Source: CAD feature listing. Evaluate the final solid. Frame: model axes, mm. Face numbers are marked on the shaded views. A direction names the side the tool comes from. Give positions to 0.01 mm unless a question says otherwise; leave off trailing zeros. Write each loop counter-clockwise with the first axis right and the second up, starting at its lowest first coordinate (ties: lowest second). Pieces come first, ordered by that corner, then holes. Notation, with made-up numbers: (31.25, 43) - (83.25, 43) arc R24 ccw to (83.25, 66) - close; hole circle Ø7 at (52, -11). An arc over 180 degrees is marked (long way). Answer as a JSON object with one key per item and string values. Group by question number.
from build123d import *

# Parameters (mm, degrees)
SKETCH1_R           = 10.85
SKETCH1_R_2         = 1.55
BOSS_EXTRUDE1_DEPTH = 7
CUT_EXTRUDE1_DEPTH  = 10
SKETCH3_R           = 1.55
BOSS_EXTRUDE2_DEPTH = 2.5
SKETCH6_W           = 5.995922228
SKETCH6_H           = 11.403727684
CUT_EXTRUDE3_DEPTH  = 11.5
CHAMFER2_SIZE       = 1
SKETCH7_R           = 1.5
CUT_EXTRUDE4_DEPTH  = 11.5
CHAMFER3_SIZE       = 0.5


with BuildPart() as part:
    # Sketch1 → Boss-Extrude1 (new body)
    with BuildSketch(Plane.XY):
        Circle(SKETCH1_R)
        with Locations((-7.8, 0)):
            Circle(SKETCH1_R_2, mode=Mode.SUBTRACT)
        with Locations(Location((7.8, 0, 0), (0, 0, 180))):
            Circle(SKETCH1_R_2, mode=Mode.SUBTRACT)
    extrude(amount=BOSS_EXTRUDE1_DEPTH)

    # Sketch2 → Cut-Extrude1 (cut)
    with BuildSketch(Plane.XY.offset(7)):
        with BuildLine():
            Line((-2.214560219, -5.749305929), (-2.214560219, -7.027203312))
            ThreePointArc((-2.214560219, -7.027203312), (-1.775220391, -8.087863484), (-0.714560219, -8.527203312))
            Line((-0.714560219, -8.527203312), (0.714560219, -8.527203312))
            ThreePointArc((0.714560219, -8.527203312), (1.775220391, -8.087863484), (2.214560219, -7.027203312))
            Line((2.214560219, -7.027203312), (2.214560219, -5.749305929))
            ThreePointArc((2.214560219, -5.749305929), (2.4555074, -3.56735999), (3.166737835, -1.490560796))
            ThreePointArc((3.166737835, -1.490560796), (3.5, 0), (3.166737835, 1.490560796))
            ThreePointArc((3.166737835, 1.490560796), (2.4555074, 3.56735999), (2.214560219, 5.749305929))
            Line((2.214560219, 5.749305929), (2.214560219, 8.304826852))
            ThreePointArc((2.214560219, 8.304826852), (1.775220391, 9.365487023), (0.714560219, 9.804826852))
            Line((0.714560219, 9.804826852), (-0.714560219, 9.804826852))
            ThreePointArc((-0.714560219, 9.804826852), (-1.775220391, 9.365487023), (-2.214560219, 8.304826852))
            Line((-2.214560219, 8.304826852), (-2.214560219, 5.749305929))
            ThreePointArc((-2.214560219, 5.749305929), (-2.4555074, 3.56735999), (-3.166737835, 1.490560796))
            ThreePointArc((-3.166737835, 1.490560796), (-3.5, 0), (-3.166737835, -1.490560796))
            ThreePointArc((-3.166737835, -1.490560796), (-2.4555074, -3.56735999), (-2.214560219, -5.749305929))
        make_face()
    extrude(amount=-CUT_EXTRUDE1_DEPTH, mode=Mode.SUBTRACT)

    # Sketch3 → Boss-Extrude2 (add)
    with BuildSketch(Plane(origin=(0, 0, 0), x_dir=(-1, 0, 0), z_dir=(0, 0, -1))):
        with Locations((-7.8, 0)):
            Circle(SKETCH3_R)
        with Locations((7.8, 0)):
            Circle(SKETCH3_R)
    extrude(amount=-BOSS_EXTRUDE2_DEPTH)

    # Sketch6 → Cut-Extrude3 (cut)
    with BuildSketch(Plane.XY.offset(7)):
        with Locations((0, 5.701863842)):
            Rectangle(SKETCH6_W, SKETCH6_H)
    extrude(amount=-CUT_EXTRUDE3_DEPTH, mode=Mode.SUBTRACT)

    # Chamfer2
    # the kernel refuses this chamfer: 1, 0.808160216 mm, written as the material it takes off along each edge
    with BuildSketch(Plane(origin=(-2.997961114, 10.427594601, 9.571682988), x_dir=(-0.9503340771083855, -0.3112316530922798, 0), z_dir=(0, 0, -1))) as chamfer2_piece_1:
        with BuildLine():
            Line((0.792665793, 0), (CHAMFER2_SIZE * 0.311231653092, -CHAMFER2_SIZE * 0.950334077108))
            Line((CHAMFER2_SIZE * 0.311231653092, -CHAMFER2_SIZE * 0.950334077108), (0, 0))
            ThreePointArc((0, 0), (0.405362345, 0.007237358), (0.792665793, 0))
        make_face()
    extrude(amount=12.143365976, mode=Mode.SUBTRACT)
    with BuildSketch(Plane(origin=(2.997961114, 10.427594601, 9.571682988), x_dir=(0.950334077108385, -0.31123165309228096, 0), z_dir=(0, 0, -1))) as chamfer2_piece_2:
        with BuildLine():
            Line((0.792665793, 0), (CHAMFER2_SIZE * 0.311231653092, CHAMFER2_SIZE * 0.950334077108))
            Line((CHAMFER2_SIZE * 0.311231653092, CHAMFER2_SIZE * 0.950334077108), (0, 0))
            ThreePointArc((0, 0), (0.405362345, -0.007237358), (0.792665793, 0))
        make_face()
    extrude(amount=12.143365976, mode=Mode.SUBTRACT)

    # Sketch7 → Cut-Extrude4 (cut)
    with BuildSketch(Plane.XY.offset(7)):
        with Locations((-5.907204398, 5.907204398)):
            Circle(SKETCH7_R)
        with Locations((5.907204398, -5.907204398)):
            Circle(SKETCH7_R)
    extrude(amount=-CUT_EXTRUDE4_DEPTH, mode=Mode.SUBTRACT)

    # Chamfer3
    chamfer3_edges = [part.edges().sort_by_distance(p)[0] for p in [
        (-7.407204398, 5.907204398, 0),
        (4.407204398, -5.907204398, 0),
    ]]
    chamfer(chamfer3_edges, length=CHAMFER3_SIZE)


solid = part.part
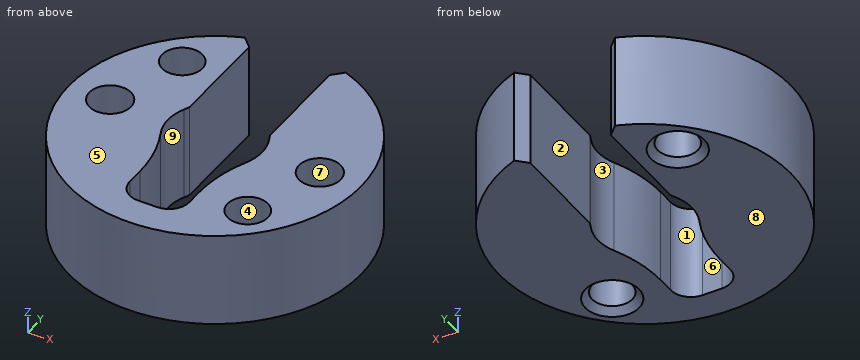
Q1. Section D-D on y = 3. Return the cut outline in (x, z).
Q2. Ray query, probe 1 along X at (y, z) = (7, 5); probe 2 along X at (y, z) = (6, 5.25); probe 3 along X at (y, z) = (2, 3.25). Return the intervals inside material, ascending. Write a range as [from, to].
Q3. Section B-B on z = 1.5. Return the cut outline in (x, y), then the cut area to 3 significant figures.
Q4. Section C-C on z = 4.5. Return the cut outline in (x, y), then the cut area to 3 significant figures.
Q5. First-contact query: pin 1 Ø1.8 at (x, y) = (5.91, -5.91) entering from +Z; pin 2 Ø1.5 at (x, y) = (7.5, -0.5) entering from +Z; pin 3 Ø1 at (y, z) = (-6.5, 4.5) entering from -X; pin 4 Ø0.7 at (x, z) = (0, 3) entering from +Y. Flat tips, straight axial feed; report the tip coordinate or a pass-through.
Q6. Section A-A on y = 0. Return the cut outline in (x, z), then the cut area to 3 significant figures.
Q7. Reachability of the marked faces 5, 6, 7, 8 and 9 from +Z, -Z, +X, -X, +Y, -Y: full face, straight path, thin tool, end or side. Return the list, or none.
Q8. Draft query along Y for the marked faces 1, 2, 3 and 4. Return one class per face: released by +Y, released by -Y, zero draft, split by the parting line, or undercut.
Taken from the geometry:
{
 "1": {"outline": "(-10.43, 0) - (-3, 0) - (-3, 7) - (-10.43, 7) - close; (3, 0) - (10.43, 0) - (10.43, 7) - (3, 7) - close"},
 "2": {"probe 1": "x = [-8.29, -6.93], [-4.88, -3], [3, 8.29]", "probe 2": "x = [-9.04, -7.4], [-4.41, -3], [3, 9.04]", "probe 3": "x = [-10.66, -3], [3, 10.66]"},
 "3": {"outline": "(-3.75, 10.18) arc R10.85 ccw (long way) to (3.75, 10.18) - (3, 9.43) - (3, 1.87) arc R10 ccw to (3.17, 1.49) arc R3.5 cw to (3.17, -1.49) arc R10 ccw to (2.21, -5.75) - (2.21, -7.03) arc R1.5 cw to (0.71, -8.53) - (-0.71, -8.53) arc R1.5 cw to (-2.21, -7.03) - (-2.21, -5.75) arc R10 ccw to (-3.17, -1.49) arc R3.5 cw to (-3.17, 1.49) arc R10 ccw to (-3, 1.87) - (-3, 9.43) - close; hole circle Ø3 at (-5.91, 5.91); hole circle Ø3 at (5.91, -5.91)", "area": "247 mm²"},
 "4": {"outline": "(-3.75, 10.18) arc R10.85 ccw (long way) to (3.75, 10.18) - (3, 9.43) - (3, 1.87) arc R10 ccw to (3.17, 1.49) arc R3.5 cw to (3.17, -1.49) arc R10 ccw to (2.21, -5.75) - (2.21, -7.03) arc R1.5 cw to (0.71, -8.53) - (-0.71, -8.53) arc R1.5 cw to (-2.21, -7.03) - (-2.21, -5.75) arc R10 ccw to (-3.17, -1.49) arc R3.5 cw to (-3.17, 1.49) arc R10 ccw to (-3, 1.87) - (-3, 9.43) - close; hole circle Ø3.1 at (-7.8, 0); hole circle Ø3 at (-5.91, 5.91); hole circle Ø3 at (5.91, -5.91); hole circle Ø3.1 at (7.8, 0)", "area": "231 mm²"},
 "5": {"pin 1": "passes through", "pin 2": "stops at z = 2.5", "pin 3": "stops at x = -9.04", "pin 4": "stops at y = -8.53"},
 "6": {"outline": "(-10.85, 0) - (-3.5, 0) - (-3.5, 7) - (-6.25, 7) - (-6.25, 2.5) - (-9.35, 2.5) - (-9.35, 7) - (-10.85, 7) - close; (3.5, 0) - (10.85, 0) - (10.85, 7) - (9.35, 7) - (9.35, 2.5) - (6.25, 2.5) - (6.25, 7) - (3.5, 7) - close", "area": "75.0 mm²"},
 "7": {"face 5": "+Z, +X, -X, +Y, -Y", "face 6": "+Z, -Z, +Y", "face 7": "+Z", "face 8": "-Z, +X, -X, +Y, -Y", "face 9": "+Z, -Z"},
 "8": {"face 1": "released by +Y", "face 2": "zero draft", "face 3": "undercut", "face 4": "undercut"}
}
